Read the model definition and answer for the solid it produces. Units are mm, in the model's axes. Face numbers are marked on the shaded views. A direction names the side the tool comes from. Give positions to 0.01 mm unless a question says otherwise; leave off trailing zeros. Order: outer loops, then holes, each group sorted by start corner. A loop starts at its lowest first (then second) coordinate and runs counter-clockwise, first axis right, second up.
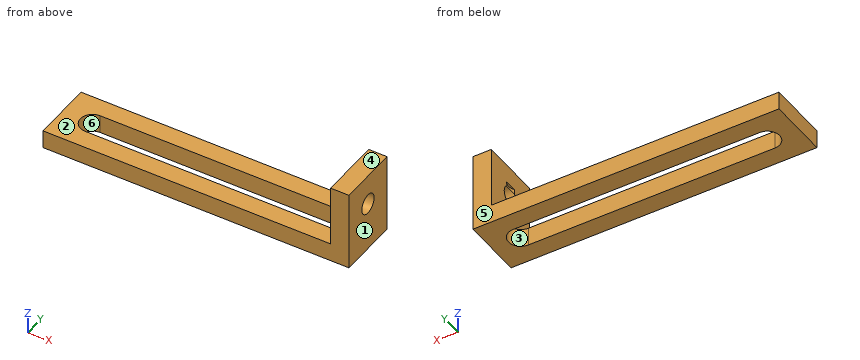
```python
from build123d import *

# Parameters (mm, degrees)
SKETCH1_W           = 50
SKETCH1_H           = 10
BOSS_EXTRUDE1_DEPTH = 3
SKETCH2_W           = 3
SKETCH2_H           = 10
BOSS_EXTRUDE2_DEPTH = 10
SKETCH3_R           = 1.614445202
CUT_EXTRUDE1_DEPTH  = 10
CUT_EXTRUDE2_DEPTH  = 10


with BuildPart() as part:
    # Sketch1 → Boss-Extrude1 (new body)
    with BuildSketch(Plane.XY):
        Rectangle(SKETCH1_W, SKETCH1_H)
    extrude(amount=BOSS_EXTRUDE1_DEPTH)

    # Sketch2 → Boss-Extrude2 (add)
    with BuildSketch(Plane.XY.offset(3)):
        with Locations((23.5, 0)):
            Rectangle(SKETCH2_W, SKETCH2_H)
    extrude(amount=BOSS_EXTRUDE2_DEPTH)

    # Sketch3 → Cut-Extrude1 (cut)
    with BuildSketch(Plane(origin=(25, 0, 0), x_dir=(0, 0, -1), z_dir=(1, 0, 0))):
        with Locations((-8, 0)):
            Circle(SKETCH3_R)
    extrude(amount=-CUT_EXTRUDE1_DEPTH, mode=Mode.SUBTRACT)

    # Sketch5 → Cut-Extrude2 (cut)
    with BuildSketch(Plane(origin=(0, 0, 0), x_dir=(-1, 0, 0), z_dir=(0, 0, -1))):
        with BuildLine():
            Line((20, -2), (-20.306358663, -2))
            ThreePointArc((-20.306358663, -2), (-22.306358663, 0), (-20.306358663, 2))
            Line((-20.306358663, 2), (20, 2))
            ThreePointArc((20, 2), (22, 0), (20, -2))
        make_face()
    extrude(amount=-CUT_EXTRUDE2_DEPTH, mode=Mode.SUBTRACT)


solid = part.part
```
1) A tool of negligible diameter and unlimited length cuts with its end or side. For the marked faces 1, 2 and 3, from which of +Z, -Z, +X, -X, +Y, -Y can it reach the whole face along a straight path? Write none if from no direction.
Final values:
face 1: +Z, -Z, +X, +Y, -Y
face 2: +Z, -X, +Y, -Y
face 3: -Z
2) The part is cut by section A-A on x = 6. Determine the outline of the cut face in (y, z).
Final values:
outline: (-5, 0) - (-2, 0) - (-2, 3) - (-5, 3) - close; (2, 0) - (5, 0) - (5, 3) - (2, 3) - close
3) The part is cut by section B-B on y = 0. Determine the outline of the cut face in (x, z).
Final values:
outline: (-25, 0) - (-22, 0) - (-22, 3) - (-25, 3) - close; (22, 10) - (22.31, 10) - (22.31, 9.61) - (25, 9.61) - (25, 13) - (22, 13) - close; (22.31, 0) - (25, 0) - (25, 6.39) - (22.31, 6.39) - close
4) Consider L1, parallel to Y at x = 6, z = 1; L2, parallel to Y at x = 23, z = 8; L3, parallel to Z at x = 23.2, y = 0. Determine where each line is inside the solid, lowest interval first.
Final values:
L1: y = -5 to -2, 2 to 5
L2: y = -5 to -1.61, 1.61 to 5
L3: z = 0 to 6.39, 9.61 to 13
5) Given pin 1 (6 mm diameter, centred on x = 12, y = -2, fed in from -Z); pin 2 (6 mm diameter, centred on x = -18.5, y = 2.5, fed in from +Z), each flat-ended and moving along its own axis, determine where each tip first touches the part or whether it passes through.
Final values:
pin 1: stops at z = 0
pin 2: stops at z = 3
6) For a pull along Y with two mould halves and no side action, classify the marked faces 4, 5 and 6 as released by +Y, released by -Y, zero draft, split by the parting line, or undercut.
Final values:
face 4: zero draft
face 5: released by +Y
face 6: undercut
7) The part is cut by section D-D on z = 4.75. Determine the outline of the cut face in (x, y), and give its area (3 significant figures).
Final values:
outline: (22, -5) - (25, -5) - (25, 5) - (22, 5) - (22, 1.06) arc R2 cw to (22, -1.06) - close
area: 29.6 mm2
8) The part is cut by section C-C on z = 8. Determine the outline of the cut face in (x, y), and give its area (3 significant figures).
Final values:
outline: (22, -5) - (25, -5) - (25, -1.61) - (22, -1.61) - close; (22, 1.61) - (25, 1.61) - (25, 5) - (22, 5) - close
area: 20.3 mm2
